Check sheet for the modelled part. Datum: model origin and axes. Units: mm. Face numbers are marked on the shaded views. A direction names the side the tool comes from. Round coordinates to 2 decimals unless told otherwise and drop trailing zeros. Write each loop counter-clockwise with the first axis right and the second up, starting at its lowest first coordinate (ties: lowest second). Pieces come first, ordered by that corner, then holes. Notation, with made-up numbers: (30.5, 56) -> (79.5, 56) arc R25 ccw to (79.5, 94) -> close; hole circle Ø5 at (47.5, -14). An arc over 180 degrees is marked (long way). One line per item, written item: value.
from build123d import *

# Parameters (mm, degrees)
BOSS_EXTRUDE1_DEPTH = 170
BOSS_EXTRUDE2_DEPTH = 1.5


with BuildPart() as part:
    # Sketch1 → Boss-Extrude1 (new body)
    with BuildSketch(Plane.XY):
        with BuildLine():
            Line((69.5, 140.5), (-69.5, 140.5))
            ThreePointArc((-69.5, 140.5), (-71.267766953, 139.767766953), (-72, 138))
            Line((-72, 138), (-72, -138))
            ThreePointArc((-72, -138), (-71.267766953, -139.767766953), (-69.5, -140.5))
            Line((-69.5, -140.5), (69.5, -140.5))
            ThreePointArc((69.5, -140.5), (71.267766953, -139.767766953), (72, -138))
            Line((72, -138), (72, 138))
            ThreePointArc((72, 138), (71.267766953, 139.767766953), (69.5, 140.5))
        make_face()
        with BuildLine():
            Line((-69.5, -139), (69.5, -139))
            ThreePointArc((69.5, -139), (70.207106781, -138.707106781), (70.5, -138))
            Line((70.5, -138), (70.5, 138))
            ThreePointArc((70.5, 138), (70.207106781, 138.707106781), (69.5, 139))
            Line((69.5, 139), (-69.5, 139))
            ThreePointArc((-69.5, 139), (-70.207106781, 138.707106781), (-70.5, 138))
            Line((-70.5, 138), (-70.5, -138))
            ThreePointArc((-70.5, -138), (-70.207106781, -138.707106781), (-69.5, -139))
        make_face(mode=Mode.SUBTRACT)
    extrude(amount=BOSS_EXTRUDE1_DEPTH)

    # Sketch2 → Boss-Extrude2 (add)
    with BuildSketch(Plane.XY.offset(170)):
        with BuildLine():
            Line((-69.5, -140.5), (69.5, -140.5))
            ThreePointArc((69.5, -140.5), (71.267766953, -139.767766953), (72, -138))
            Line((72, -138), (72, 138))
            ThreePointArc((72, 138), (71.267766953, 139.767766953), (69.5, 140.5))
            Line((69.5, 140.5), (-69.5, 140.5))
            ThreePointArc((-69.5, 140.5), (-71.267766953, 139.767766953), (-72, 138))
            Line((-72, 138), (-72, -138))
            ThreePointArc((-72, -138), (-71.267766953, -139.767766953), (-69.5, -140.5))
        make_face()
    extrude(amount=BOSS_EXTRUDE2_DEPTH)


solid = part.part
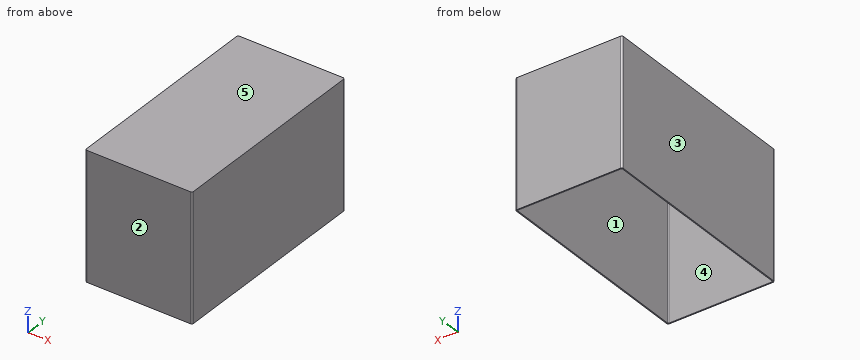
Item 1: Sectioned sample at A-A (z = 32). Enter the section's corners in (x, y), then the cut area to 3 significant figures.
Result set:
outline: (-72, -138) arc R2.5 ccw to (-69.5, -140.5) -> (69.5, -140.5) arc R2.5 ccw to (72, -138) -> (72, 138) arc R2.5 ccw to (69.5, 140.5) -> (-69.5, 140.5) arc R2.5 ccw to (-72, 138) -> close; hole (-70.5, -138) arc R1 ccw to (-69.5, -139) -> (69.5, -139) arc R1 ccw to (70.5, -138) -> (70.5, 138) arc R1 ccw to (69.5, 139) -> (-69.5, 139) arc R1 ccw to (-70.5, 138) -> close
area: 1,260 mm^2
Item 2: Tool access check on the marked faces 1 and 2. Record the directions out of +Z, -Z, +X, -X, +Y, -Y that give a thin tool (end or side, any length) a straight path to the whole face; none if there is none.
Result set:
face 1: -Z
face 2: +Z, -Z, +X, -X, -Y
Item 3: Release check for a two-part mould opening along X. For the marked faces 3, 4 and 5 record: pulls with the +X half, pulls with the -X half, needs draft (parallel to the pull), parting line crosses it, or undercut.
Result set:
face 3: pulls with the -X half
face 4: undercut
face 5: needs draft
Item 4: Material ranges on line 1 along Y through (x, z) = (-4, 153); line 2 along X through (y, z) = (-30, 140); line 3 along Z through (x, y) = (5.5, -48), recorded low to high.
Result set:
line 1: -140.5 to -139, 139 to 140.5
line 2: -72 to -70.5, 70.5 to 72
line 3: 170 to 171.5
Item 5: Sectioned sample at B-B (x = -17.5). Enter the section's corners in (y, z), then the cut area to 4 significant figures.
Result set:
outline: (-140.5, 0) -> (-139, 0) -> (-139, 170) -> (139, 170) -> (139, 0) -> (140.5, 0) -> (140.5, 171.5) -> (-140.5, 171.5) -> close
area: 931.5 mm^2
Item 6: Sectioned sample at C-C (y = -53.5). Enter the section's corners in (x, z).
Result set:
outline: (-72, 0) -> (-70.5, 0) -> (-70.5, 170) -> (70.5, 170) -> (70.5, 0) -> (72, 0) -> (72, 171.5) -> (-72, 171.5) -> close
